from build123d import *

# Parameters (mm, degrees)
F1_DEPTH = 7.62
F2_R     = 3.17499
F4_R     = 1.016
F5_DEPTH = 7.62
F3_R     = 1.016
F6_DEPTH = 7.62


# Not quite as in the source:
# - a fillet or chamfer is up to 0.001 mm smaller than in the source, because OpenCascade refuses the exact size


with BuildPart() as f1:
    # F0 (on Right) → F1 (new body)
    with BuildSketch(Plane.YZ):
        Polygon((50.292, -3.175), (50.292, 3.175), (0, 3.175), (-50.292, 3.175), (-50.292, -3.175), align=None)
    extrude(amount=F1_DEPTH)

    # F2 (radius 3.175 in the source; OpenCascade refuses exactly that, so slightly less here)
    f2_edges = [f1.edges().sort_by_distance(p)[0] for p in [
        (7.62, 0, -3.175),
        (7.62, 0, 3.175),
    ]]
    fillet(f2_edges, radius=F2_R)

    # F4 (on face) → F5 (cut)
    with BuildSketch(Plane.XZ.offset(50.292)):
        with Locations((3.81, 0)):
            Circle(F4_R)
    extrude(amount=-F5_DEPTH, mode=Mode.SUBTRACT)

    # F3 (on face) → F6 (cut)
    with BuildSketch(Plane(origin=(0, 50.292, 0), x_dir=(-1, 0, 0), z_dir=(0, 1, 0))):
        with Locations((-3.81, 0)):
            Circle(F3_R)
    extrude(amount=-F6_DEPTH, mode=Mode.SUBTRACT)


solid = f1.part
The listing builds one solid part. Answer for the finished solid, in the listing's coordinates (mm). A direction names the side the tool comes from. Round coordinates to 2 decimals unless told otherwise and drop trailing zeros. Order: outer loops, then holes, each group sorted by start corner. A loop starts at its lowest first (then second) coordinate and runs counter-clockwise, first axis right, second up. Notation, with made-up numbers: (-28, 39.25) - (14, 39.25) arc R17 cw to (14, 50.25) - close; hole circle Ø4 at (74.25, -25). An arc over 180 degrees is marked (long way). Write item = value, one per line. Start each with the question number.
1) Section B-B, the plane x = 6 is taken. Write down the section's boundary in (y, z), plus the area to 3 significant figures.
2) For a pull along Z with two mould halves and no side action, classify faces 1 (the flat face through (4, 42.672, 0)), 2 (the cylindrical face through (4.779, -46.535, 0.305)), 3 (the flat face through (3, -50.292, -1)), 4 (the flat face through (2, -1, -3.175)) as released by +Z, released by -Z, zero draft, split by the parting line, or undercut.
3) Given pin 1 (1.2 mm diameter, centred on x = 3.81, z = 0, fed in from +Y); pin 2 (1 mm diameter, centred on y = 4, z = -2, fed in from +X), each flat-ended and moving along its own axis, determine where each tip first touches the part or whether it passes through.
4) Straight lines are drawn through the part: L1, parallel to Z at x = 3.81, y = 47 (3 decimals); L2, parallel to Y at x = 3, z = 0; L3, parallel to X at y = -3, z = -1. For each, find the intervals that lie inside material, in ascending order.
5) For faces 5 (the flat face through (3, 50.292, 1)), 6 (the cylindrical face through (4.825, 46.535, 0.045)), 7 (the flat face through (4, -42.672, 0)), determine the directions among +Z, -Z, +X, -X, +Y, -Y from which every point of the face is accessible in a straight line to the end or side of a thin tool.
Results list:
q1.outline = (-50.29, -2.77) - (50.29, -2.77) - (50.29, 2.77) - (-50.29, 2.77) - close
q1.area = 557 mm^2
q2.face_1 = undercut
q2.face_2 = undercut
q2.face_3 = zero draft
q2.face_4 = released by -Z
q3.pin_1 = 42.67
q3.pin_2 = 7.24
q4.L1 = -3.175 to -1.016, 1.016 to 3.175
q4.L2 = -42.67 to 42.67
q4.L3 = 0 to 7.46
q5.face_5 = +Z, -Z, +X, -X, +Y
q5.face_6 = +Y
q5.face_7 = -Y
